```python
from build123d import *

# Parameters (mm, degrees)
SKETCH_1_W      = 6.5
SKETCH_1_H      = 6
EXTRUDE_1_DEPTH = 3.5
SKETCH_1_3_R    = 1.8
EXTRUDE_2_DEPTH = 6
EXTRUDE_START   = 3.5
SKETCH_1_4_R    = 0.5
EXTRUDE_3_DEPTH = 0.3
EXTRUDE_START_2 = -1
SKETCH_2_W      = 0.8
SKETCH_2_H      = 0.3
EXTRUDE_4_DEPTH = 5


with BuildPart() as part:
    # 草图1 → 凸台-拉伸1 (new body)
    with BuildSketch(Plane(origin=(0, 0, 0), x_dir=(1, 0, 0), z_dir=(0, 1, 0))):
        Rectangle(SKETCH_1_W, SKETCH_1_H)
    extrude(amount=EXTRUDE_1_DEPTH)

    # 草图1<3> → 凸台-拉伸2 (add)
    with BuildSketch(Plane(origin=(0, 0, 0), x_dir=(1, 0, 0), z_dir=(0, 1, 0))):
        with Locations(Location((0, 0, 0), (0, 0, 90))):
            Circle(SKETCH_1_3_R)
    extrude(amount=EXTRUDE_2_DEPTH)

    # 草图1<4> → 凸台-拉伸3 (add)
    with BuildSketch(Plane(origin=(0, 0, 0), x_dir=(1, 0, 0), z_dir=(0, 1, 0)).offset(EXTRUDE_START)):
        with Locations(Location((-2.275, 2.1, 0), (0, 0, 90))):
            Circle(SKETCH_1_4_R)
        with Locations(Location((-2.275, -2.1, 0), (0, 0, 90))):
            Circle(SKETCH_1_4_R)
        with Locations(Location((2.275, -2.1, 0), (0, 0, 90))):
            Circle(SKETCH_1_4_R)
        with Locations(Location((2.275, 2.1, 0), (0, 0, 90))):
            Circle(SKETCH_1_4_R)
    extrude(amount=EXTRUDE_3_DEPTH)

    # 草图2 → 凸台-拉伸4 (add)
    with BuildSketch(Plane.XZ.offset(EXTRUDE_START_2)):
        with Locations((-2.85, 3.15)):
            Rectangle(SKETCH_2_W, SKETCH_2_H)
        with Locations((2.85, 3.15)):
            Rectangle(SKETCH_2_W, SKETCH_2_H)
        with Locations((-2.85, -3.15)):
            Rectangle(SKETCH_2_W, SKETCH_2_H)
        with Locations((2.85, -3.15)):
            Rectangle(SKETCH_2_W, SKETCH_2_H)
    extrude(amount=EXTRUDE_4_DEPTH)


solid = part.part
```
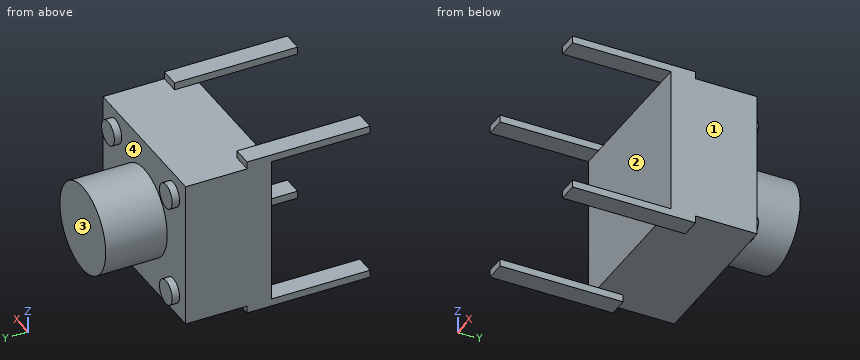
Work out the finished part from the listing and answer in its coordinate system (mm). Face numbers are marked on the shaded views. A direction names the side the tool comes from. Round coordinates to 2 decimals unless told otherwise and drop trailing zeros. Loops run counter-clockwise (first coordinate to the right, second up) from the corner with the lowest first, then second, coordinate; pieces in that order, holes last. Notation, with made-up numbers: M 83.25,-1.5 L 95.25,-1.5 A14 cw 95.25,12.5 Z; hole C 18.25,12 d5. An arc over 180 degrees is marked long. One line per question, with ' | ' between items.
Q1. Consider line 1 along Y through (x, z) = (-2, 1.5); line 2 along Y through (x, z) = (0.25, 0.25); line 3 along Z through (x, y) = (-3, 2.5). Determine where each line is inside the solid, lowest interval first. Write a range as from..to.
Conclusion:
line 1: y = 0..3.5 | line 2: y = 0..6 | line 3: z = -3..3
Q2. Find section D-D, the plane z = 2.1. Give the vertices of the cut face in (x, y) (3 decimals), then the cut area to 4 significant figures.
Conclusion:
outline: M -3.25,0 L 3.25,0 L 3.25,3.5 L 2.775,3.5 L 2.775,3.8 L 1.775,3.8 L 1.775,3.5 L -1.775,3.5 L -1.775,3.8 L -2.775,3.8 L -2.775,3.5 L -3.25,3.5 Z | area: 23.35 mm2
Q3. Find section B-B, the plane z = 0. Give the vertices of the cut face in (x, y), then the cut area to 4 significant figures.
Conclusion:
outline: M -3.25,0 L 3.25,0 L 3.25,3.5 L 1.8,3.5 L 1.8,6 L -1.8,6 L -1.8,3.5 L -3.25,3.5 Z | area: 31.75 mm2
Q4. Find section A-A, the plane y = -3. Give the vertices of the cut face in (x, z), then the cut area to 3 significant figures.
Conclusion:
outline: M -3.25,-3.3 L -2.45,-3.3 L -2.45,-3 L -3.25,-3 Z; M -3.25,3 L -2.45,3 L -2.45,3.3 L -3.25,3.3 Z; M 2.45,-3.3 L 3.25,-3.3 L 3.25,-3 L 2.45,-3 Z; M 2.45,3 L 3.25,3 L 3.25,3.3 L 2.45,3.3 Z | area: 0.960 mm2
Q5. A tool of negligible diameter and unlimited length cuts with its end or side. For the marked faces 3 and 4, from which of +Z, -Z, +X, -X, +Y, -Y can it reach the whole face along a straight path? Write none if from no direction.
Conclusion:
face 3: +Z, -Z, +X, -X, +Y | face 4: +Y
Q6. Each of these flat-tipped pins is pushed along its axis until it touches: pin 1 Ø1 at (x, y) = (2, 3) entering from +Z; pin 2 Ø2 at (x, z) = (2.5, 1) entering from -Y; pin 3 Ø0.5 at (x, z) = (2.5, -2) entering from +Y. Where does it stop, or does it pass through?
Conclusion:
pin 1: stops at z = 3 | pin 2: stops at y = 0 | pin 3: stops at y = 3.8
Q7. The mould has two halves that part along Z. Classify the marked faces 1 and 2: +Z half, -Z half, draft (parallel to the pull), parting line (faces both ways), or undercut.
Conclusion:
face 1: draft | face 2: undercut
Q8. Find section C-C, the plane x = -0.75. Give the vertices of the cut face in (y, z), then the cut area to 3 significant figures.
Conclusion:
outline: M 0,-3 L 3.5,-3 L 3.5,-1.64 L 6,-1.64 L 6,1.64 L 3.5,1.64 L 3.5,3 L 0,3 Z | area: 29.2 mm2
